```python
from build123d import *

# Parameters (mm, degrees)
CROQUIS1_R              = 1.25
SALIENTE_EXTRUIR1_DEPTH = 12
CORTAR_EXTRUIR1_DEPTH   = 0.5


with BuildPart() as part:
    # Croquis1 → Saliente-Extruir1 (new body)
    with BuildSketch(Plane(origin=(0, 0, 0), x_dir=(1, 0, 0), z_dir=(0, 1, 0))):
        Circle(CROQUIS1_R)
    extrude(amount=SALIENTE_EXTRUIR1_DEPTH)

    # Croquis2 one side → Revolución1 (revolve)
    with BuildSketch(Plane(origin=(0, 0, 0), x_dir=(0, 0, -1), z_dir=(1, 0, 0))):
        Polygon((0, 13.25), (0, 12), (1.25, 12), (2.5, 13.25), align=None)
    revolve(axis=Axis((0, 13.25, 0), (0, -1, 0)))

    # Croquis3 → Cortar-Extruir1 (cut)
    with BuildSketch(Plane(origin=(0, 13.25, 0), x_dir=(1, 0, 0), z_dir=(0, 1, 0))):
        Polygon((1.443375673, 0), (0.721687836, 1.25), (-0.721687836, 1.25), (-1.443375673, 0), (-0.721687836, -1.25), (0.721687836, -1.25), align=None)
    extrude(amount=-CORTAR_EXTRUIR1_DEPTH, mode=Mode.SUBTRACT)

    # Croquis4 one side → Revolución2 (revolve)
    with BuildSketch(Plane.XY):
        Polygon((0, 0), (0, -1), (1.25, 0), align=None)
    revolve(axis=Axis((0, 0, 0), (0, -1, 0)))


solid = part.part
```
Design review of the part built by this model. Coordinates are the model's own, in mm. Give positions to 0.01 mm unless a question says otherwise; leave off trailing zeros. Loops run counter-clockwise (first coordinate to the right, second up) from the corner with the lowest first, then second, coordinate; pieces in that order, holes last. Notation, with made-up numbers: (11.25, 44.25) -> (39.25, 44.25) arc R31 cw to (39.25, 69.25) -> close; hole circle Ø8 at (-33.75, 87.5). An arc over 180 degrees is marked (long way). One line per item, written item: value.
Q1. We need section A-A on y = 1.5. Give the boundary of the cut face in (x, z), and give its area (3 significant figures).
Numbers:
outline: circle Ø2.5 at (0, 0)
area: 4.91 mm^2
Q2. Draft analysis for pull direction Z (two halves, no side actions). For faces 1 (the flat face through (0, 12.75, 0)), 2 (the cylindrical face through (-0.27, 5.92, 1.22)), 3 (the flat face through (-1.1, 13.25, -1.1)), state which applies: pulls with the +Z half, pulls with the -Z half, needs draft (parallel to the pull), parting line crosses it, or undercut.
Numbers:
face 1: undercut
face 2: parting line crosses it
face 3: needs draft
Q3. For L1, parallel to X at y = 12.5, z = -0.4; L2, parallel to Z at x = 0.75, y = 12.25; L3, parallel to Y at x = -1.8, z = -0.5, list the stretches that pass through material, from the lowest coordinate up.
Numbers:
L1: x = -1.7 to 1.7
L2: z = -1.3 to 1.3
L3: y = 12.62 to 13.25
Q4. For pin 1 Ø3 at (x, z) = (0, 0.5) entering from +Y; pin 2 Ø0.6 at (x, y) = (0.5, 13) entering from -Z, all flat-tipped, find the tip position at first contact; note any pin that passes through.
Numbers:
pin 1: stops at y = 13.25
pin 2: stops at z = -2.48
